Can you work these out from the model? Positions are in its coordinate system, mm. Face numbers are marked on the shaded views. A direction names the side the tool comes from. Coordinates: 2 decimals unless noted, no trailing zeros. Loops run counter-clockwise (first coordinate to the right, second up) from the corner with the lowest first, then second, coordinate; pieces in that order, holes last.
```python
from build123d import *

# Parameters (mm, degrees)
F0_W      = 12.5476
F0_H      = 22.6568
F1_DEPTH  = 22.4282
F3_W      = 12.5476
F3_H      = 22.6568
F3_H_2    = 4.8768
F4_DEPTH  = 2.4765
F6_DEPTH  = 4.2672
F7_R      = 3.3909
F8_DEPTH  = 5.334
F10_DEPTH = 1.4732


with BuildPart() as f1:
    # F0 (on Top) → F1 (new body)
    with BuildSketch(Plane.XY):
        Rectangle(F0_W, F0_H)
    extrude(amount=F1_DEPTH)

    # F3 (on offset) → F4 (join)
    with BuildSketch(Plane.XY.offset(17.9832)):
        Rectangle(F3_W, F3_H)
        with Locations((0, -13.7668)):
            Rectangle(F3_W, F3_H_2)
        with Locations((0, 13.7668)):
            Rectangle(F3_W, F3_H_2)
    extrude(amount=-F4_DEPTH)

    # F5 (on face) → F6 (join)
    with BuildSketch(Plane.XY.offset(22.4282)):
        with BuildLine():
            ThreePointArc((-6.2738, 5.0546), (0, -1.2192), (6.2738, 5.0546))
            ThreePointArc((6.2738, 5.0546), (4.4362465254, 9.4908465222), (4.5e-09, 11.3284))
            ThreePointArc((4.5e-09, 11.3284), (-4.4362465222, 9.4908465254), (-6.2738, 5.0546))
        make_face()
    extrude(amount=F6_DEPTH)

    # F7 (on face) → F8 (join)
    with BuildSketch(Plane.XY.offset(26.6954)):
        with Locations((0, 5.0546)):
            Circle(F7_R)
    extrude(amount=F8_DEPTH)

    # F9 (on face) → F10 (join)
    with BuildSketch(Plane.XY.offset(32.0294)):
        with BuildLine():
            Line((3.3909, 5.0546), (3.3323728486, 4.4273089926))
            ThreePointArc((3.3323728486, 4.4273089926), (3.376236507, 4.7395922876), (3.3909, 5.0546))
        make_face()
        with BuildLine():
            Line((1.905, -10.8712), (3.3323728486, 4.4273089926))
            Line((3.3323728486, 4.4273089926), (3.3909, 5.0546))
            Line((3.3909, 5.0546), (3.3323728486, 5.6818910074))
            Line((3.3323728486, 5.6818910074), (1.905, 20.9804))
            ThreePointArc((1.905, 20.9804), (0, 22.8854), (-1.905, 20.9804))
            Line((-1.905, 20.9804), (-3.3323728486, 5.6818910074))
            Line((-3.3323728486, 5.6818910074), (-3.3909, 5.0546))
            Line((-3.3909, 5.0546), (-3.3323728486, 4.4273089926))
            Line((-3.3323728486, 4.4273089926), (-1.905, -10.8712))
            ThreePointArc((-1.905, -10.8712), (0, -12.7762), (1.905, -10.8712))
        make_face()
        with BuildLine():
            Line((3.3323728486, 5.6818910074), (3.3909, 5.0546))
            ThreePointArc((3.3909, 5.0546), (3.376236507, 5.3696077124), (3.3323728486, 5.6818910074))
        make_face()
        with BuildLine():
            ThreePointArc((-3.3909, 5.0546), (-3.376236507, 4.7395922876), (-3.3323728486, 4.4273089926))
            Line((-3.3323728486, 4.4273089926), (-3.3909, 5.0546))
        make_face()
        with BuildLine():
            ThreePointArc((-3.3323728486, 5.6818910074), (-3.376236507, 5.3696077124), (-3.3909, 5.0546))
            Line((-3.3909, 5.0546), (-3.3323728486, 5.6818910074))
        make_face()
    extrude(amount=-F10_DEPTH)


solid = f1.part
```
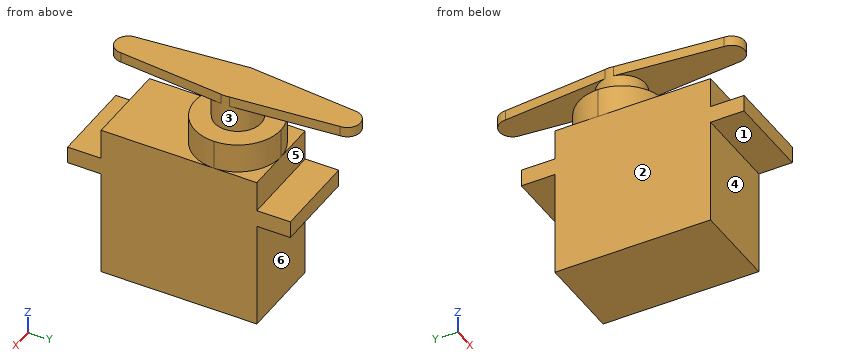
(1) I want a section at D-D on y = -10. Write out the boundary of the cut face in (x, z).
Check values:
outline: (-6.27, 0) - (6.27, 0) - (6.27, 22.43) - (-6.27, 22.43) - close; (-1.99, 30.56) - (1.99, 30.56) - (1.99, 32.03) - (-1.99, 32.03) - close
(2) Which directions (+Z, -Z, +X, -X, +Y, -Y) give clear straight access to the entire face, cutting with the end or side of a thin tool? Please do the marked faces 4, 5 and 6.
Check values:
face 4: -Z, +X, -X, -Y
face 5: +X, -X, +Y
face 6: -Z, +X, -X, +Y
(3) If we mould it in two halves opening along Z, with no side actions, what happens to the marked faces 1, 2 and 3? For each: released by +Z, released by -Z, zero draft, split by the parting line, or undercut.
Check values:
face 1: released by -Z
face 2: zero draft
face 3: undercut
(4) I want a section at A-A on y = -0.5. Write out the boundary of the cut face in (x, z).
Check values:
outline: (-6.27, 0) - (6.27, 0) - (6.27, 22.43) - (2.92, 22.43) - (2.92, 26.7) - (-2.92, 26.7) - (-2.92, 22.43) - (-6.27, 22.43) - close; (-2.87, 30.56) - (2.87, 30.56) - (2.87, 32.03) - (-2.87, 32.03) - close
(5) If I drill on probe 1 along Z at (x, y) = (0, -9); probe 2 along Y at (x, z) = (-1, 22); probe 3 along Z at (x, y) = (-0.5, 0.5), over which ranges is the centre line in solid material (lowest first)?
Check values:
probe 1: z = 0 to 22.43, 30.56 to 32.03
probe 2: y = -11.33 to 11.33
probe 3: z = 0 to 26.7, 30.56 to 32.03
(6) I'm going to push flat-ended pins straight in: pin 1 (2 mm diameter, centred on x = -2.5, y = -9.5, fed in from +Z); pin 2 (1.2 mm diameter, centred on x = 2, z = 17, fed in from +Y); pin 3 (6.5 mm diameter, centred on x = -2.5, z = 9.5, fed in from -Y); pin 4 (1 mm diameter, centred on x = 3.5, z = 6, fed in from +Y). Where does each tip first touch, or does it pass through?
Check values:
pin 1: stops at z = 32.03
pin 2: stops at y = 16.21
pin 3: stops at y = -11.33
pin 4: stops at y = 11.33
(7) I want a section at B-B on x = -5.5. Write out the boundary of the cut face in (y, z), then the cut area to 3 significant figures.
Check values:
outline: (-16.21, 15.51) - (-11.33, 15.51) - (-11.33, 0) - (11.33, 0) - (11.33, 15.51) - (16.21, 15.51) - (16.21, 17.98) - (11.33, 17.98) - (11.33, 22.43) - (8.07, 22.43) - (8.07, 26.7) - (2.04, 26.7) - (2.04, 22.43) - (-11.33, 22.43) - (-11.33, 17.98) - (-16.21, 17.98) - close
area: 558 mm2
(8) I want a section at C-C on z = 8.5. Write out the boundary of the cut face in (x, y).
Check values:
outline: (-6.27, -11.33) - (6.27, -11.33) - (6.27, 11.33) - (-6.27, 11.33) - close
